Autodesk Inventor part; units mm, degrees
ref_plane "YZ Plane" through (0, 0, 0) normal (1, 0, 0) x (0, 1, 0)
ref_plane "XZ Plane" through (0, 0, 0) normal (0, 1, 0) x (-1, 0, 0)
ref_plane "XY Plane" through (0, 0, 0) normal (0, 0, 1) x (1, 0, 0)
sketch "Sketch1" plane through (0, 0, 0) normal (0, 1, 0) x (-1, 0, 0)
  line L0 (0, 0) -> (30, 0)
  line L1 (30, 0) -> (30, -30)
  line L2 (30, -30) -> (0, -30)
  line L3 (0, -30) -> (0, 0)
  dimension "d0" = 30
  dimension "d1" = 30
extrude "Extrusion1" add sketch "Sketch1" along normal blind 55.4
sketch "Sketch2" plane through (0, 55.4, 0) normal (0, 1, 0) x (1, 0, 0)
  line L0 (0, 0) -> (0, 30)
  line L1 (0, 0) -> (0, 4.5)
  line L2 (0, 4.5) -> (-4.5, 4.5)
  line L3 (-4.5, 4.5) -> (-25.5, 4.5)
  line L4 (-25.5, 4.5) -> (-25.5, 25.5)
  line L5 (-25.5, 25.5) -> (-4.5, 25.5)
  line L6 (-4.5, 25.5) -> (-4.5, 4.5)
  dimension "d4" = 4.5
  dimension "d5" = 4.5
  dimension "d6" = 21
  dimension "d7" = 21
extrude "Extrusion2" cut sketch "Sketch2" against normal blind 30
sketch "Sketch3" plane through (0, 0, 0) normal (0, -1, 0) x (1, 0, 0)
  line L0 (0, 0) -> (-15, 0)
  line L1 (0, 0) -> (-30, 0)
  line L2 (-15, 0) -> (-15, -15)
  circle A0 centre (-15, -15) radius 2
  dimension "d10" = 15
  dimension "d11" = 4
extrude "Extrusion3" cut sketch "Sketch3" against normal blind 5
fillet "Fillet1" radius 5 4 edges at (0, 0, -15) (-15, 0, 0) (-15, 0, -30) (-30, 0, -15)
fillet "Fillet2" radius 5 8 edges at (-1.4645, 1.4645, -28.5355) (0, 30.2, -30) (-1.4645, 1.4645, -1.4645) (0, 30.2, 0) (-28.5355, 1.4645, -28.5355) (-30, 30.2, -30) (-28.5355, 1.4645, -1.4645) (-30, 30.2, 0)
properties part number "1in_2020_Endcap"
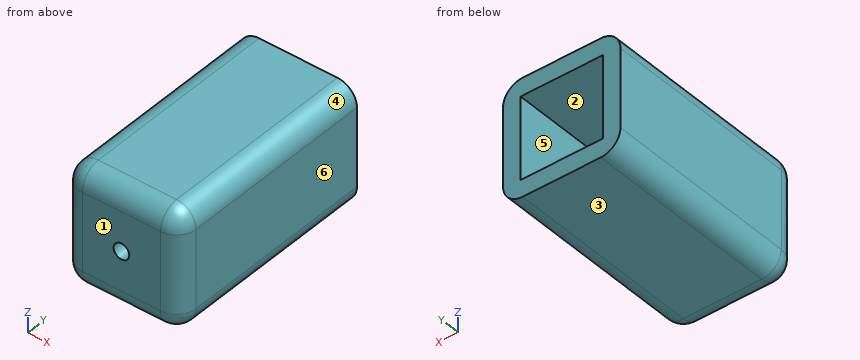
Verification items for the finished model (mm, model axes). Face numbers are marked on the shaded views. A direction names the side the tool comes from. Round coordinates to 2 decimals unless told otherwise and drop trailing zeros. Write each loop counter-clockwise with the first axis right and the second up, starting at its lowest first coordinate (ties: lowest second). Pieces come first, ordered by that corner, then holes. Notation, with made-up numbers: (-26.5, 86.5) -> (20.5, 86.5) arc R11 ccw to (20.5, 90.5) -> close; hole circle Ø2 at (63, 58.25). An arc over 180 degrees is marked (long way). Write each question's results on one line, items separated by ' | '.
Q1. Draft check along Z on the marked faces 1, 2, 3 and 4. Enter one of: released by +Z, released by -Z, zero draft, split by the parting line, or undercut.
Derived:
face 1: zero draft | face 2: undercut | face 3: released by -Z | face 4: released by +Z
Q2. Go/stop test with flat-tipped pins: pin 1 Ø6.5 at (x, z) = (-11.5, -17) entering from +Y; pin 2 Ø3 at (x, z) = (-15, -15) entering from -Y. Record where each tip stops, or that it passes through.
Derived:
pin 1: stops at y = 25.4 | pin 2: stops at y = 5
Q3. Access from +Z, -Z, +X, -X, +Y, -Y to the whole of each face (thin tool, end or side, straight path). Record for the marked faces 5 and 6.
Derived:
face 5: +Y | face 6: +Z, -Z, +X, +Y, -Y
Q4. Sectioned sample at A-A, the plane y = 44.5. Record the boundary of the cut face in (x, z).
Derived:
outline: (-30, -25) arc R5 ccw to (-25, -30) -> (-5, -30) arc R5 ccw to (0, -25) -> (0, -5) arc R5 ccw to (-5, 0) -> (-25, 0) arc R5 ccw to (-30, -5) -> close; hole (-25.5, -25.5) -> (-4.5, -25.5) -> (-4.5, -4.5) -> (-25.5, -4.5) -> close
Q5. Sectioned sample at C-C, the plane z = -19.5. Record the boundary of the cut face in (x, y).
Derived:
outline: (-30, 5) arc R5 ccw to (-25, 0) -> (-5, 0) arc R5 ccw to (0, 5) -> (0, 55.4) -> (-4.5, 55.4) -> (-4.5, 25.4) -> (-25.5, 25.4) -> (-25.5, 55.4) -> (-30, 55.4) -> close
Q6. Sectioned sample at D-D, the plane y = 15. Record the boundary of the cut face in (x, z), and give its area (3 significant figures).
Derived:
outline: (-30, -25) arc R5 ccw to (-25, -30) -> (-5, -30) arc R5 ccw to (0, -25) -> (0, -5) arc R5 ccw to (-5, 0) -> (-25, 0) arc R5 ccw to (-30, -5) -> close | area: 879 mm²
Q7. Sectioned sample at B-B, the plane x = -23.75. Record the boundary of the cut face in (y, z), and give its area (3 significant figures).
Derived:
outline: (0, -25) arc R5 ccw to (5, -30) -> (55.4, -30) -> (55.4, -25.5) -> (25.4, -25.5) -> (25.4, -4.5) -> (55.4, -4.5) -> (55.4, 0) -> (5, 0) arc R5 ccw to (0, -5) -> close | area: 1,020 mm²
Q8. Thickness scan on probe 1 along X at (y, z) = (44, -10); probe 2 along Y at (x, z) = (-6.5, -7.5). Record the ranges inside material, lowest first.
Derived:
probe 1: x = -30 to -25.5, -4.5 to 0 | probe 2: y = 0 to 25.4
